```python
from build123d import *

# Parameters (mm, degrees)
SKETCH1_W           = 52
SKETCH1_H           = 35.5
BOSS_EXTRUDE1_DEPTH = 11.6
SHELL1_T            = -1.5
SKETCH2_W           = 71.75
SKETCH2_H           = 11.6
BOSS_EXTRUDE2_DEPTH = 3.9
SKETCH3_W           = 71.75
SKETCH3_H           = 11.75
BOSS_EXTRUDE3_DEPTH = 4
FILLET1_R           = 5
SKETCH4_R           = 2.15
CUT_EXTRUDE1_DEPTH  = 41.741110994
SKETCH5_R           = 2.2
CUT_EXTRUDE2_DEPTH  = 52.786345932


with BuildPart() as part:
    # Sketch1 → Boss-Extrude1 (new body)
    with BuildSketch(Plane(origin=(0, 0, 0), x_dir=(1, 0, 0), z_dir=(0, 1, 0))):
        Rectangle(SKETCH1_W, SKETCH1_H)
    extrude(amount=BOSS_EXTRUDE1_DEPTH)

    # Shell1
    shell1_openings = [part.faces().sort_by_distance(p)[0] for p in [
        (0, 11.6, 0),
    ]]
    offset(amount=SHELL1_T, openings=shell1_openings, kind=Kind.INTERSECTION)

    # Sketch2 → Boss-Extrude2 (add)
    with BuildSketch(Plane.XY.offset(17.75)):
        with Locations((0, 5.8)):
            Rectangle(SKETCH2_W, SKETCH2_H)
    extrude(amount=-BOSS_EXTRUDE2_DEPTH)

    # Sketch3 → Boss-Extrude3 (add)
    with BuildSketch(Plane.XZ):
        with Locations((0, -0.275)):
            Rectangle(SKETCH3_W, SKETCH3_H)
    extrude(amount=-BOSS_EXTRUDE3_DEPTH)

    # Fillet1
    fillet1_edges = [part.edges().sort_by_distance(p)[0] for p in [
        (-35.875, 2, 5.6),
        (35.875, 2, -6.15),
        (-35.875, 2, -6.15),
        (35.875, 2, 5.6),
    ]]
    fillet(fillet1_edges, radius=FILLET1_R)

    # Sketch4 → Cut-Extrude1 (cut, through all)
    with BuildSketch(Plane(origin=(0, 4, 0), x_dir=(1, 0, 0), z_dir=(0, 1, 0))):
        with Locations(Location((-29.825, 0.275, 0), (0, 0, 270))):
            Circle(SKETCH4_R)
        with Locations(Location((29.825, 0.275, 0), (0, 0, 270))):
            Circle(SKETCH4_R)
    extrude(amount=-CUT_EXTRUDE1_DEPTH, mode=Mode.SUBTRACT)

    # Sketch5 → Cut-Extrude2 (cut, through all)
    with BuildSketch(Plane.XY.offset(17.75)):
        with Locations((-30.075, 7.75)):
            Circle(SKETCH5_R)
        with Locations((30.075, 7.75)):
            Circle(SKETCH5_R)
    extrude(amount=-CUT_EXTRUDE2_DEPTH, mode=Mode.SUBTRACT)


solid = part.part
```
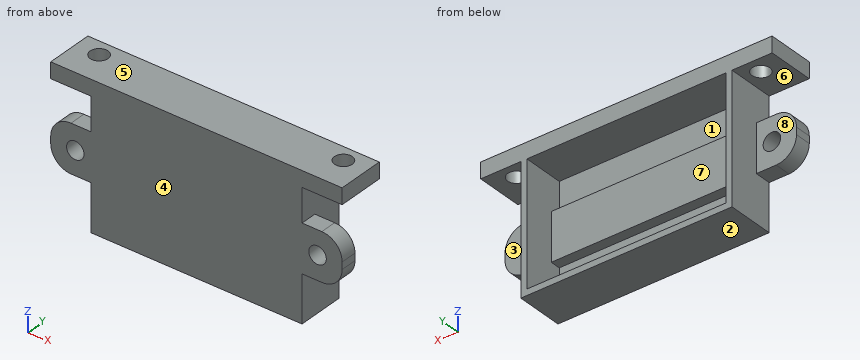
The listing builds one solid part. Answer for the finished solid, in the listing's coordinates (mm). Face numbers are marked on the shaded views. A direction names the side the tool comes from. Give positions to 0.01 mm unless a question says otherwise; leave off trailing zeros. Loops run counter-clockwise (first coordinate to the right, second up) from the corner with the lowest first, then second, coordinate; pieces in that order, holes last. Notation, with made-up numbers: M 77.5,-23.5 L 107.5,-23.5 A17 cw 107.5,2.5 Z; hole C 19.25,-39 d10. An arc over 180 degrees is marked long. One line per item, written item: value.
1. Section A-A on y = 7.75 is taken. Determine the outline of the cut face in (x, z) (3 decimals), plus the area to 3 significant figures.
Found:
outline: M -35.875,13.85 L -32.275,13.85 L -32.275,17.75 L -35.875,17.75 Z; M -27.875,13.85 L -26,13.85 L -26,-17.75 L 26,-17.75 L 26,13.85 L 27.875,13.85 L 27.875,17.75 L -27.875,17.75 Z; M 32.275,13.85 L 35.875,13.85 L 35.875,17.75 L 32.275,17.75 Z; hole M -24.5,-16.25 L 24.5,-16.25 L 24.5,13.85 L -24.5,13.85 Z
area: 414 mm^2
2. Section C-C on x = -3 is taken. Determine the outline of the cut face in (y, z).
Found:
outline: M 0,-17.75 L 11.6,-17.75 L 11.6,-16.25 L 1.5,-16.25 L 1.5,-6.15 L 4,-6.15 L 4,5.6 L 1.5,5.6 L 1.5,13.85 L 11.6,13.85 L 11.6,17.75 L 0,17.75 Z
3. For a pull along Z with two mould halves and no side action, classify the marked faces 1, 2 and 3 as pulls with the +Z half, pulls with the -Z half, needs draft (parallel to the pull), parting line crosses it, or undercut.
Found:
face 1: undercut
face 2: pulls with the -Z half
face 3: needs draft
4. Section D-D on y = 3 is taken. State how many separate pieces and enclosed holes the cut face has, plus the area to 3 significant figures.
Found:
separate pieces: 1
enclosed holes: 4
area: 1,210 mm^2
5. Each of these flat-tipped pins is pushed along its axis until it touches: P1, Ø3, axis at x = -2, z = -14, coming from the +Y side; P2, Ø3.5, axis at x = -30.075, y = 7.75, coming from the -Z side; P3, Ø3, axis at y = 7, z = -5, coming from the +X side; P4, Ø6.5, axis at x = 7, z = 8.5, coming from the +Y side. Where does it stop, or does it pass through?
Found:
P1: y = 1.5
P2: through
P3: x = 26
P4: y = 4
6. Section B-B on z = -9 is taken. Determine the outline of the cut face in (x, y), plus the area to 3 significant figures.
Found:
outline: M -26,0 L 26,0 L 26,11.6 L 24.5,11.6 L 24.5,1.5 L -24.5,1.5 L -24.5,11.6 L -26,11.6 Z
area: 108 mm^2
7. For the marked faces 4, 5, 6, 7 and 8, determine the directions among +Z, -Z, +X, -X, +Y, -Y from which every point of the face is accessible in a straight line to the end or side of a thin tool.
Found:
face 4: +Z, -Z, +X, -X, -Y
face 5: +Z, +X, -X, +Y, -Y
face 6: -X, +Y, -Y
face 7: +Y
face 8: -Z, -X, +Y
8. Find the intervals of material crossed by probe 1 along Z at (x, y) = (-2.5, 2.75); probe 2 along X at (y, z) = (6.5, -4); probe 3 along Z at (x, y) = (16, 6.5), in increasing order.
Found:
probe 1: -17.75 to -16.25, -6.15 to 5.6, 13.85 to 17.75
probe 2: -26 to -24.5, 24.5 to 26
probe 3: -17.75 to -16.25, 13.85 to 17.75
